Read the model definition and answer for the solid it produces. Units are mm, in the model's axes. A direction names the side the tool comes from. Round coordinates to 2 decimals unless told otherwise and drop trailing zeros. Order: outer loops, then holes, each group sorted by start corner. A loop starts at its lowest first (then second) coordinate and runs counter-clockwise, first axis right, second up. Notation, with made-up numbers: (40, -7) -> (77, -7) arc R22 ccw to (77, 9) -> close; hole circle Ø3 at (62, -9.5). An arc over 180 degrees is marked (long way). Answer as a JSON object with one key per item and string values. Group by question number.
Item 1: Consider probe 1 along X at (y, z) = (6.5, -2.25); probe 2 along Y at (x, z) = (-13, -4.25) (3 decimals); probe 3 along Y at (x, z) = (36.5, 5.75) (3 decimals). Determine where each line is inside the solid, lowest interval first. Write a range as from..to.
Item 2: Given P1, Ø1.5, axis at x = -23, z = 4, coming from the -Y side; P2, Ø12, axis at x = -16, z = -3, coming from the +Y side (3 decimals); P3, Ø5, axis at x = -19, y = 3.5, coming from the -Z side; P4, Ø0.8, axis at x = 40, z = -14.5, coming from the +Y side, each flat-ended and moving along its own axis, determine where each tip first touches the part or whether it passes through.
Item 3: Section D-D, the plane z = 3.75 is taken. Write down the section's boundary in (x, y) (3 decimals).
Item 4: Section C-C, the plane y = 28.5 is taken. Write down the section's boundary in (x, z).
Item 5: For faces 5 (the flat face through (29, 0, -4)), 6 (the flat face through (34.801, 21, -4)), 7 (the cylindrical face through (-33.376, 28.592, 5.797)), determine the directions among +Z, -Z, +X, -X, +Y, -Y from which every point of the face is accessible in a straight line to the end or side of a thin tool.
Item 6: The mould has two halves that part along Z. Classify faces 1 (the cylindrical face through (38.633, 28.592, 5.797)), 2 (the flat face through (7, 2, 8.391)), 3 (the flat face through (-37.208, 20, -4)), 4 (the flat face through (7, 2, -17.009)): pulls with the +Z half, pulls with the -Z half, needs draft (parallel to the pull), parting line crosses it, or undercut.
Item 7: Section B-B, the plane x = 10.5 is taken. Write down the section's boundary in (y, z) (3 decimals), plus the area to 3 significant figures.
Item 8: Section A-A, the plane y = 6 is taken. Write down the section's boundary in (x, z).
from build123d import *

# Parameters (mm, degrees)
SKETCH1_W           = 69.85
SKETCH1_H           = 25.4
BOSS_EXTRUDE1_DEPTH = 3.175
SKETCH2_W           = 3.937
SKETCH2_H           = 25.4
BOSS_EXTRUDE2_DEPTH = 35.56
SKETCH6_R           = 1.5875
CUT_EXTRUDE1_DEPTH  = 35.56
SKETCH10_W          = 25.4
SKETCH10_H          = 38.735
BOSS_EXTRUDE3_DEPTH = 6.096
SKETCH11_W          = 25.4
SKETCH11_H          = 38.735
BOSS_EXTRUDE4_DEPTH = 6.096
SKETCH14_R          = 1.25
CUT_EXTRUDE2_DEPTH  = 20.574
SKETCH15_W          = 21.082
SKETCH15_H          = 25.4
SKETCH15_R          = 1.5875
BOSS_EXTRUDE6_DEPTH = 3.175


with BuildPart() as part:
    # Sketch1 → Boss-Extrude1 (new body)
    with BuildSketch(Plane(origin=(0, 0, 0), x_dir=(1, 0, 0), z_dir=(0, 1, 0))):
        with Locations((3.81330156, 4.308535529)):
            Rectangle(SKETCH1_W, SKETCH1_H)
    extrude(amount=BOSS_EXTRUDE1_DEPTH)

    # Sketch2 → Boss-Extrude2 (add)
    with BuildSketch(Plane(origin=(0, 3.175, 0), x_dir=(1, 0, 0), z_dir=(0, 1, 0))):
        with Locations((-29.14319844, 4.308535529)):
            Rectangle(SKETCH2_W, SKETCH2_H)
        with Locations((36.76980156, 4.308535529)):
            Rectangle(SKETCH2_W, SKETCH2_H)
    extrude(amount=BOSS_EXTRUDE2_DEPTH)

    # Sketch6 → Cut-Extrude1 (cut)
    with BuildSketch(Plane.XZ):
        with Locations((-3.55269844, -6.340535529)):
            Circle(SKETCH6_R)
        with Locations((11.17930156, -6.340535529)):
            Circle(SKETCH6_R)
    extrude(amount=-CUT_EXTRUDE1_DEPTH, mode=Mode.SUBTRACT)

    # Sketch10 → Boss-Extrude3 (add)
    with BuildSketch(Plane.ZY.offset(31.11169844)):
        with Locations((-4.308535529, 19.3675)):
            Rectangle(SKETCH10_W, SKETCH10_H)
    extrude(amount=BOSS_EXTRUDE3_DEPTH)

    # Sketch11 → Boss-Extrude4 (add)
    with BuildSketch(Plane(origin=(38.73830156, 0, 0), x_dir=(0, 0, -1), z_dir=(1, 0, 0))):
        with Locations((4.308535529, 19.3675)):
            Rectangle(SKETCH11_W, SKETCH11_H)
    extrude(amount=BOSS_EXTRUDE4_DEPTH)

    # Sketch14 → Cut-Extrude2 (cut)
    with BuildSketch(Plane(origin=(0, 38.735, 0), x_dir=(1, 0, 0), z_dir=(0, 1, 0))):
        with Locations((-32.12769844, 14.468535529)):
            Circle(SKETCH14_R)
        with Locations((-32.12769844, -5.851464471)):
            Circle(SKETCH14_R)
        with Locations((39.88130156, 14.468535529)):
            Circle(SKETCH14_R)
        with Locations((39.88130156, -5.851464471)):
            Circle(SKETCH14_R)
    extrude(amount=-CUT_EXTRUDE2_DEPTH, mode=Mode.SUBTRACT)

    # Sketch15 → Boss-Extrude6 (add)
    with BuildSketch(Plane.XZ):
        with Locations((3.81330156, -4.308535529)):
            Rectangle(SKETCH15_W, SKETCH15_H)
        with Locations((-3.55269844, -6.340535529)):
            Circle(SKETCH15_R, mode=Mode.SUBTRACT)
        with Locations((11.17930156, -6.340535529)):
            Circle(SKETCH15_R, mode=Mode.SUBTRACT)
    extrude(amount=BOSS_EXTRUDE6_DEPTH)


solid = part.part
Values found:
{
 "1": {"probe 1": "-37.21..-27.17, 34.8..44.83", "probe 2": "0..3.175", "probe 3": "0..38.735"},
 "2": {"P1": "y = 0", "P2": "y = 3.175", "P3": "z = -17.01", "P4": "y = 18.16"},
 "3": {"outline": "(-37.208, 0) -> (-6.728, 0) -> (-6.728, -3.175) -> (14.354, -3.175) -> (14.354, 0) -> (44.834, 0) -> (44.834, 38.735) -> (34.801, 38.735) -> (34.801, 3.175) -> (-27.175, 3.175) -> (-27.175, 38.735) -> (-37.208, 38.735) -> close"},
 "4": {"outline": "(-37.21, -17.01) -> (-27.17, -17.01) -> (-27.17, 8.39) -> (-37.21, 8.39) -> close; (34.8, -17.01) -> (44.83, -17.01) -> (44.83, 8.39) -> (34.8, 8.39) -> close; hole circle Ø2.5 at (-32.13, -14.47); hole circle Ø2.5 at (-32.13, 5.85); hole circle Ø2.5 at (39.88, -14.47); hole circle Ø2.5 at (39.88, 5.85)"},
 "5": {"face 5": "+Z, -Z, +X, -Y", "face 6": "+Z, -Z, +Y", "face 7": "+Y"},
 "6": {"face 1": "undercut", "face 2": "pulls with the +Z half", "face 3": "needs draft", "face 4": "pulls with the -Z half"},
 "7": {"outline": "(-3.175, -17.009) -> (3.175, -17.009) -> (3.175, -7.775) -> (-3.175, -7.775) -> close; (-3.175, -4.906) -> (3.175, -4.906) -> (3.175, 8.391) -> (-3.175, 8.391) -> close", "area": "143 mm2"},
 "8": {"outline": "(-37.21, -17.01) -> (-27.17, -17.01) -> (-27.17, 8.39) -> (-37.21, 8.39) -> close; (34.8, -17.01) -> (44.83, -17.01) -> (44.83, 8.39) -> (34.8, 8.39) -> close"}
}
